Design review of the part shown in the three views and the two pictorial views. Dimensions are in mm from the part's minimum x, y and z. Coordinates: 2 decimals unless noted, no trailing zeros. Write each loop counter-clockwise with the first axis right and the second up, starting at its lowest first coordinate (ties: lowest second). Pieces come first, ordered by that corner, then holes. Notation, with made-up numbers: (-20.75, 61.5) -> (34.25, 61.5) arc R15 ccw to (34.25, 87.5) -> close; hole circle Ø7 at (71.25, 83). An arc over 180 degrees is marked (long way). Answer in a Markdown table with one row per item. Add a question column.
Item 1: Take a section at B-B, the plane x = 63. Give the number of separate pieces and of enclosed holes in the cut face, and give its area (3 significant figures).
Item 2: Clearance check with flat-ended pins moving along their axes: P1, Ø1, axis at x = 79.5, z = 1.5, coming from the +Y side (3 decimals); P2, Ø1, axis at x = 24.5, z = 2.5, coming from the -Y side (3 decimals). State where each tip first meets the part, or that it passes through.
Item 3: Take a section at A-A, the plane y = 45.5. Write out the cut boundary in (x, z) (1 decimal).
Item 4: Take a section at D-D, the plane x = 51.5. Write out the cut boundary in (y, z) (1 decimal).
Item 5: To check wall thickness, follow line 1 (Y direction, x = 64, z = 2.1); line 2 (X direction, y = 21.5, z = 2.65) (1 decimal); line 3 (X direction, y = 3.5, z = 2.85) (1 decimal). State the ranges of each line that lie inside material, in increasing order.
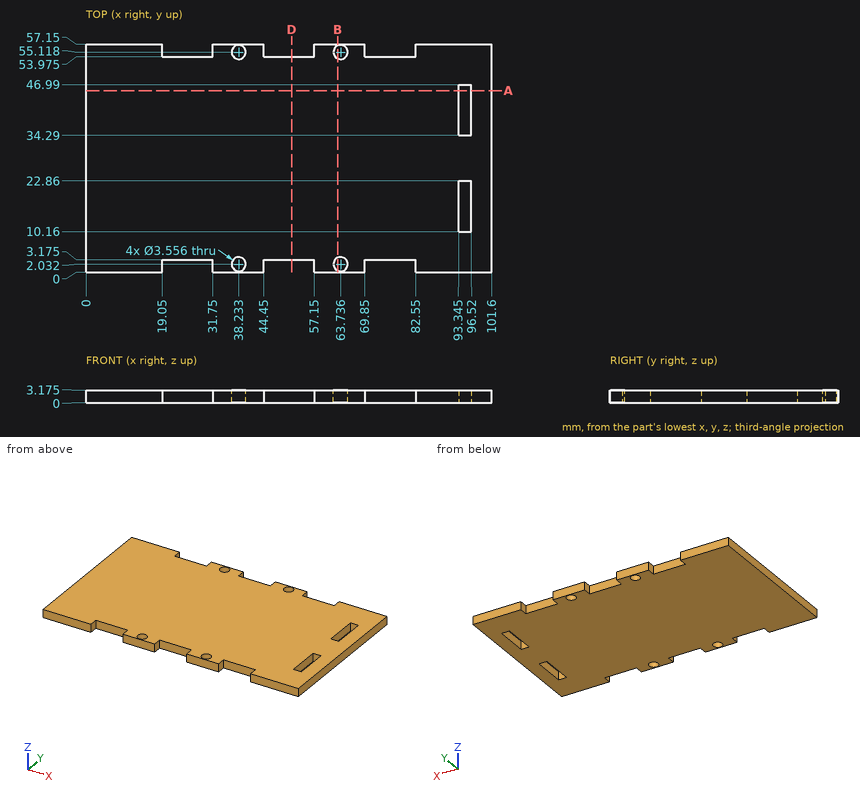
Answers:
| question | item | result |
|---|---|---|
| 1 | separate pieces | 3 |
| 1 | enclosed holes | 0 |
| 1 | area | 161 mm^2 |
| 2 | P1 | stops at y = 53.975 |
| 2 | P2 | stops at y = 3.175 |
| 3 | outline | (0, 0) -> (93.3, 0) -> (93.3, 3.2) -> (0, 3.2) -> close; (96.5, 0) -> (101.6, 0) -> (101.6, 3.2) -> (96.5, 3.2) -> close |
| 4 | outline | (3.2, 0) -> (54, 0) -> (54, 3.2) -> (3.2, 3.2) -> close |
| 5 | line 1 | y = 0 to 0.27, 3.79 to 53.36, 56.88 to 57.15 |
| 5 | line 2 | x = 0 to 93.3, 96.5 to 101.6 |
| 5 | line 3 | x = 0 to 37.2, 39.2 to 62.7, 64.7 to 101.6 |
